```python
from build123d import *

# Parameters (mm, degrees)
SKETCH2_R           = 1.55
BOSS_EXTRUDE1_DEPTH = 12.35
SKETCH3_R           = 1.5


with BuildPart() as part:
    # Sketch2 → Boss-Extrude1 (new body)
    with BuildSketch(Plane(origin=(0, 0, 0), x_dir=(1, 0, 0), z_dir=(0, 1, 0))):
        with BuildLine():
            ThreePointArc((-39.917771177, -2.56350234), (-39.988230838, 0.970254828), (-39.746472283, 4.496436488))
            Line((-39.746472283, 4.496436488), (-46.205274029, 5.227107417))
            ThreePointArc((-46.205274029, 5.227107417), (-46.34972481, 3.735372816), (-46.44602765, 2.239757921))
            ThreePointArc((-46.44602765, 2.239757921), (-48.2434435, -0.585642563), (-46.591633685, -3.498564803))
            Line((-46.591633685, -3.498564803), (-39.917771177, -2.56350234))
        make_face()
        with Locations(Location((-44.994489261, -0.668082567, 0), (0, 0, 270))):
            Circle(SKETCH2_R, mode=Mode.SUBTRACT)
    extrude(amount=BOSS_EXTRUDE1_DEPTH)

    # Sweep1: sweep along a path in Sketch7
    with BuildLine(Plane(origin=(0, 0, 0), x_dir=(1, 0, 0), z_dir=(0, 1, 0))) as sweep1_path:
        ThreePointArc((-39.746472283, 4.496436488), (-33.564183671, 21.758804529), (-20.329010289, 34.448967193))
    # Sketch3 → Sweep1 (sweep)
    with BuildSketch(Plane(origin=(0, 0, 0), x_dir=(-0.9936618070654342, 0, -0.11241091219030289), z_dir=(0.11241091219030287, 0, -0.993661807065434))):
        with Locations((43.4, 9.175)):
            Circle(SKETCH3_R)
        with Locations((43.4, 3.175)):
            Circle(SKETCH3_R)
    sweep(path=sweep1_path.line)


solid = part.part
```
Could you check a few things on this model? Use its own coordinates, in mm. Round coordinates to 2 decimals unless told otherwise and drop trailing zeros. Write each loop counter-clockwise with the first axis right and the second up, starting at its lowest first coordinate (ties: lowest second). Pieces come first, ordered by that corner, then holes. Notation, with made-up numbers: M 65,86.5 L 112,86.5 A26 ccw 112,102.5 Z; hole C 10.25,20 d2. An arc over 180 degrees is marked long. Answer in a Markdown table with one row per item. Add a question column.
Q1. Imagine slicing it at A-A (y = 10). Please give me the cut outline in (x, z), then the cut area to 3 significant figures.
Q2. Will these pins go through, and if not, where does the flat tip stop? pin 1 Ø1.5 at (y, z) = (1.5, -29) entering from -X; pin 2 Ø5 at (y, z) = (11, -11.5) entering from +X; pin 3 Ø4 at (y, z) = (8, -3.5) entering from -X.
Q3. If we mould it in two halves opening along Z, with no side actions, what happens to faces 1 (the flat face through (-44, 0, -1)), 2 (the flat face through (-22.07, 9.15, -37.4)), 3 (the flat face through (-42.931, 6.089, -4.857))? For each: +Z half, -Z half, draft (parallel to the pull), parting line (faces both ways), or undercut.
Q4. Imagine slicing it at B-B (y = 2.25). Please give me the cut outline in (x, z).
Q5. Imagine slicing it at C-C (y = 5.25). Please give me the cut outline in (x, z).
Q6. If I drill on line 1 (Y direction, x = -25.25, z = -36); line 2 (Z direction, x = -41.5, y = 10.75); line 3 (X direction, y = 2.5, z = -18), over which ranges is the centre line in solid material (lowest first)? Write a range as from..to.
Values:
| question | item | result |
|---|---|---|
| 1 | outline | M -46.59,3.5 A3.25 ccw -46.45,-2.24 A46.5 ccw -46.21,-5.23 L -44.37,-5.02 A44.65 ccw -22.69,-38.46 L -21.42,-36.3 A42.15 cw -41.88,-4.74 L -39.75,-4.5 A40 cw -39.92,2.56 Z; hole C -44.99,0.67 d3.1 |
| 1 | area | 152 mm^2 |
| 2 | pin 1 | x = -34.07 |
| 2 | pin 2 | x = -39.7 |
| 2 | pin 3 | x = -47.42 |
| 3 | face 1 | draft |
| 3 | face 2 | -Z half |
| 3 | face 3 | undercut |
| 4 | outline | M -46.59,3.5 A3.25 ccw -46.45,-2.24 A46.5 ccw -46.21,-5.23 L -44.3,-5.01 A44.58 ccw -22.66,-38.39 L -21.46,-36.36 A42.22 cw -41.95,-4.75 L -39.75,-4.5 A40 cw -39.92,2.56 Z; hole C -44.99,0.67 d3.1 |
| 5 | outline | M -46.59,3.5 A3.25 ccw -46.45,-2.24 A46.5 ccw -46.21,-5.23 L -39.75,-4.5 A40 cw -39.92,2.56 Z; hole C -44.99,0.67 d3.1 |
| 6 | line 1 | 1.79..4.56, 7.79..10.56 |
| 6 | line 2 | -4.69..2.79 |
| 6 | line 3 | -40.96..-38.01 |
